from build123d import *

# Parameters (mm, degrees)
SKETCH1_W                      = 50
SKETCH1_H                      = 35
SKETCH1_R                      = 8.5
BOSS_EXTRUDE1_DEPTH            = 8
F_3_0MM_DOWEL_HOLE1_AT_2_COUNT = 2
F_3_0MM_DOWEL_HOLE1_AT_2_PITCH = 40.311288741
CBORE_FOR_M5_SHCS1_AT_2_COUNT  = 2
CBORE_FOR_M5_SHCS1_AT_2_PITCH  = 40.311288741
SKETCH6_R                      = 11.5
CUT_EXTRUDE1_DEPTH             = 1.5
CHAMFER1_SIZE                  = 1
CHAMFER2_SIZE                  = 0.2


with BuildPart() as part:
    # Sketch1 → Boss-Extrude1 (new body)
    with BuildSketch(Plane(origin=(0, 0, 0), x_dir=(1, 0, 0), z_dir=(0, 1, 0))):
        Rectangle(SKETCH1_W, SKETCH1_H)
        with Locations(Location((0, 0, 0), (0, 0, 270))):
            Circle(SKETCH1_R, mode=Mode.SUBTRACT)
    extrude(amount=BOSS_EXTRUDE1_DEPTH)

    # Sketch3 → Ø3.0mm Dowel Hole1 (revolve, cut)
    with BuildSketch(Plane(origin=(-17.5, 8, -10), x_dir=(0, 0, 1), z_dir=(1, 0, 0))):
        Polygon((0, 0), (0, 8), (1.75, 8), (1.5, 7.75), (1.5, 0.25), (1.75, 0), align=None)
    f_3_0mm_dowel_hole1 = revolve(axis=Axis((-17.5, 14.35, -10), (0, -1, 0)), mode=Mode.SUBTRACT)

    # Ø3.0mm Dowel Hole1 at 2: Ø3.0mm Dowel Hole1 ×2
    with Locations(*[Vector(0.8682431421244593, 0, 0.49613893835683387) * (i * F_3_0MM_DOWEL_HOLE1_AT_2_PITCH) for i in range(1, F_3_0MM_DOWEL_HOLE1_AT_2_COUNT)]):
        add(f_3_0mm_dowel_hole1, mode=Mode.SUBTRACT)

    # Sketch5 → CBORE for M5 SHCS1 (revolve, cut)
    with BuildSketch(Plane(origin=(17.5, 8, -10), x_dir=(0, 0, 1), z_dir=(1, 0, 0))):
        Polygon((0, 0), (0, 8), (3, 8), (2.75, 7.75), (2.75, 5.25), (3, 5), (5, 5), (5, 0.25), (5.25, 0), align=None)
    cbore_for_m5_shcs1 = revolve(axis=Axis((17.5, 14.35, -10), (0, -1, 0)), mode=Mode.SUBTRACT)

    # CBORE for M5 SHCS1 at 2: CBORE for M5 SHCS1 ×2
    with Locations(*[Vector(-0.8682431421244593, 0, 0.49613893835683387) * (i * CBORE_FOR_M5_SHCS1_AT_2_PITCH) for i in range(1, CBORE_FOR_M5_SHCS1_AT_2_COUNT)]):
        add(cbore_for_m5_shcs1, mode=Mode.SUBTRACT)

    # Sketch6 → Cut-Extrude1 (cut)
    with BuildSketch(Plane(origin=(0, 0, 0), x_dir=(1, 0, 0), z_dir=(0, 1, 0))):
        with Locations(Location((0, 0, 0), (0, 0, 270))):
            Circle(SKETCH6_R)
    extrude(amount=CUT_EXTRUDE1_DEPTH, mode=Mode.SUBTRACT)

    # Chamfer1
    chamfer1_edges = [part.edges().sort_by_distance(p)[0] for p in [
        (-25, 4, -17.5),
        (25, 4, -17.5),
        (25, 4, 17.5),
        (-25, 4, 17.5),
    ]]
    chamfer(chamfer1_edges, length=CHAMFER1_SIZE)

    # Chamfer2
    chamfer2_edges = [part.edges().sort_by_distance(p)[0] for p in [
        (0, 8, -8.5),
        (0, 1.5, -8.5),
        (0, 0, -11.5),
        (0, 0, -17.5),
        (0, 8, -17.5),
        (-25, 0, 0),
        (25, 0, 0),
        (0, 0, 17.5),
        (-24.5, 0, 17),
        (-24.5, 0, -17),
        (24.5, 0, 17),
        (24.5, 0, -17),
        (25, 8, 0),
        (-25, 8, 0),
        (0, 8, 17.5),
        (-24.5, 8, 17),
        (-24.5, 8, -17),
        (24.5, 8, 17),
        (24.5, 8, -17),
    ]]
    chamfer(chamfer2_edges, length=CHAMFER2_SIZE)


solid = part.part
Design review of the part built by this model. Coordinates are the model's own, in mm. A direction names the side the tool comes from. Coordinates: 2 decimals unless noted, no trailing zeros. Loops run counter-clockwise (first coordinate to the right, second up) from the corner with the lowest first, then second, coordinate; pieces in that order, holes last. Notation, with made-up numbers: (7, -8.75) -> (55, -8.75) arc R9 cw to (55, 3.25) -> close; hole circle Ø10 at (-32.75, 88.5). An arc over 180 degrees is marked (long way). Use a Markdown table: item, result. Add a question column.
Item 1: The part is to be moulded in two halves that separate along X. For faces 4 (the cylindrical face through (16.67, 1.52, -7.38)), 5 (the flat face through (24.5, 3.9, -17)), 6 (the cylindrical face through (8.428, 4.707, -1.107)), 7 (the flat face through (0, 4, -17.5)), say which applies: +X half, -X half, draft (parallel to the pull), parting line (faces both ways), or undercut.
Item 2: We need section B-B, the plane z = 0. Write out the cut boundary in (x, y).
Item 3: Machinability: for faces 1 (the flat face through (20, 3, -12)), 2 (the flat face through (-25, 4, 0)), 3 (the cylindrical face through (9.7, 0.84, 6.18)), which of the approach directions +Z, -Z, +X, -X, +Y, -Y give a long, thin tool a straight path to every point of the face, cutting with its end or side? Answer none if there is none.
Item 4: We need section D-D, the plane y = 5.75. Write out the cut boundary in (x, z).
Item 5: Clearance check with a flat-ended pin moving along its axis: P1, Ø1, axis at x = -16.5, z = 7.5, coming from the +Y side. State where the tip first meets the part, or that it passes through.
Item 6: Wall thickness on L1, parallel to Z at x = 17.5, y = 6; L2, parallel to Z at x = 17.5, y = 1.3; L3, parallel to X at y = 5.55, z = 10: over which ranges is each line inside the solid? List them lowest first. Write a range as from..to.
Item 7: We need section C-C, the plane y = 1. Write out the cut boundary in (x, z).
Item 8: We need section A-A, the plane x = 17.5. Count the separate pieces of the cut face and the enclosed holes in it, and give its area (3 significant figures).
Numbers:
| question | item | result |
|---|---|---|
| 1 | face 4 | undercut |
| 1 | face 5 | +X half |
| 1 | face 6 | undercut |
| 1 | face 7 | draft |
| 2 | outline | (-25, 0.2) -> (-24.8, 0) -> (-11.7, 0) -> (-11.5, 0.2) -> (-11.5, 1.5) -> (-8.7, 1.5) -> (-8.5, 1.7) -> (-8.5, 7.8) -> (-8.7, 8) -> (-24.8, 8) -> (-25, 7.8) -> close; (8.5, 1.7) -> (8.7, 1.5) -> (11.5, 1.5) -> (11.5, 0.2) -> (11.7, 0) -> (24.8, 0) -> (25, 0.2) -> (25, 7.8) -> (24.8, 8) -> (8.7, 8) -> (8.5, 7.8) -> close |
| 3 | face 1 | +Y |
| 3 | face 2 | +Z, -Z, -X, +Y, -Y |
| 3 | face 3 | -Y |
| 4 | outline | (-25, -16.5) -> (-24, -17.5) -> (24, -17.5) -> (25, -16.5) -> (25, 16.5) -> (24, 17.5) -> (-24, 17.5) -> (-25, 16.5) -> close; hole circle Ø10 at (-17.5, 10); hole circle Ø3 at (-17.5, -10); hole circle Ø17 at (0, 0); hole circle Ø10 at (17.5, -10); hole circle Ø3 at (17.5, 10) |
| 5 | P1 | stops at y = 3 |
| 6 | L1 | z = -17.5..-15, -5..8.5, 11.5..17.5 |
| 6 | L2 | z = -17.5..-12.75, -7.25..8.5, 11.5..17.5 |
| 6 | L3 | x = -25..-22.5, -12.5..16, 19..25 |
| 7 | outline | (-25, -16.5) -> (-24, -17.5) -> (24, -17.5) -> (25, -16.5) -> (25, 16.5) -> (24, 17.5) -> (-24, 17.5) -> (-25, 16.5) -> close; hole circle Ø5.5 at (-17.5, 10); hole circle Ø3 at (-17.5, -10); hole circle Ø23 at (0, 0); hole circle Ø5.5 at (17.5, -10); hole circle Ø3 at (17.5, 10) |
| 8 | separate pieces | 3 |
| 8 | enclosed holes | 0 |
| 8 | area | 189 mm^2 |
